Part model, mm, in its own coordinate system. Face numbers are marked on the shaded views. A direction names the side the tool comes from. Give positions to 0.01 mm unless a question says otherwise; leave off trailing zeros. Write each loop counter-clockwise with the first axis right and the second up, starting at its lowest first coordinate (ties: lowest second). Pieces come first, ordered by that corner, then holes.
```python
from build123d import *

# Parameters (mm, degrees)
SKETCH_1_R          = 20
SKETCH_1_W          = 63.973509934
SKETCH_1_H          = 26
EXTRUDE_1_DEPTH     = 10
SKETCH_2_W          = 45
SKETCH_2_H          = 20
CUT_EXTRUDE_1_DEPTH = 7
SKETCH_3_R          = 10
CUT_EXTRUDE_2_DEPTH = 8
SKETCH_4_R          = 4
CUT_EXTRUDE_3_DEPTH = 7
SKETCH_6_W          = 10
SKETCH_6_H          = 8
EXTRUDE_2_DEPTH     = 15
CHAMFER_2_SIZE      = 5
EXTRUDE_3_DEPTH     = 20
SKETCH_8_W          = 10
SKETCH_8_H          = 12.77482578
EXTRUDE_4_DEPTH     = 15
SKETCH_9_W          = 7
SKETCH_9_H          = 20
EXTRUDE_5_DEPTH     = 10
SKETCH_10_W         = 7
SKETCH_10_H         = 20
EXTRUDE_6_DEPTH     = 7
SKETCH_11_W         = 10
SKETCH_11_H         = 15
CUT_EXTRUDE_5_DEPTH = 60.88841868
SKETCH_12_W         = 10
SKETCH_12_H         = 18
SKETCH_12_H_2       = 20.77482578
EXTRUDE_7_DEPTH     = 15
CUT_EXTRUDE_6_DEPTH = 15
FILLET_1_R          = 1
CHAMFER_3_SIZE      = 1
FILLET_2_R          = 2
SKETCH_14_R         = 7.5
SKETCH_14_R_2       = 4
EXTRUDE_8_DEPTH     = 2
FILLET_3_R          = 2
SKETCH_16_R         = 2.5
CUT_EXTRUDE_7_DEPTH = 3
CHAMFER_4_SIZE      = 0.5
FILLET_4_R          = 2


# Some blends are built 0.0001 mm under size
with BuildPart() as part:
    # 草图1 → 凸台-拉伸1 (new body)
    with BuildSketch(Plane(origin=(0, 0, 0), x_dir=(0, 0, -1), z_dir=(1, 0, 0))):
        with Locations((31.986754967, 0)):
            Circle(SKETCH_1_R)
        Rectangle(SKETCH_1_W, SKETCH_1_H)
    extrude(amount=EXTRUDE_1_DEPTH)

    # 草图2 → 切除-拉伸1 (cut)
    with BuildSketch(Plane(origin=(10, 0, 0), x_dir=(0, 0, -1), z_dir=(1, 0, 0))):
        with Locations((-9.486754967, 0)):
            Rectangle(SKETCH_2_W, SKETCH_2_H)
    extrude(amount=-CUT_EXTRUDE_1_DEPTH, mode=Mode.SUBTRACT)

    # 草图3 → 切除-拉伸2 (cut)
    with BuildSketch(Plane(origin=(10, 0, 0), x_dir=(0, 0, -1), z_dir=(1, 0, 0))):
        with Locations((31.986754967, 0)):
            Circle(SKETCH_3_R)
    extrude(amount=-CUT_EXTRUDE_2_DEPTH, mode=Mode.SUBTRACT)

    # 草图4 → 切除-拉伸3 (cut)
    with BuildSketch(Plane(origin=(2, 0, 0), x_dir=(0, 0, -1), z_dir=(1, 0, 0))):
        with Locations((31.986754967, 0)):
            Circle(SKETCH_4_R)
    extrude(amount=-CUT_EXTRUDE_3_DEPTH, mode=Mode.SUBTRACT)

    # 草图6 → 凸台-拉伸2 (add)
    with BuildSketch(Plane.XZ.offset(13)):
        with Locations((5, -12.788070813)):
            Rectangle(SKETCH_6_W, SKETCH_6_H)
        with Locations((5, 27.986754967)):
            Rectangle(SKETCH_6_W, SKETCH_6_H)
    extrude(amount=EXTRUDE_2_DEPTH)

    # 倒角2
    # the kernel refuses this chamfer: 5, 3.546264764 mm, written as the material it adds along each edge
    with BuildSketch(Plane(origin=(10, -13, -16.788070813), x_dir=(0, -0.6995038411281902, -0.7146288381019251), z_dir=(-1, 0, 0))) as chamfer_2_piece_1:
        with BuildLine():
            Line((3.535736125, 0), (CHAMFER_2_SIZE * 0.699503841128, CHAMFER_2_SIZE * 0.714628838102))
            Line((CHAMFER_2_SIZE * 0.699503841128, CHAMFER_2_SIZE * 0.714628838102), (0, 0))
            ThreePointArc((0, 0), (1.768947181, 0.07828713), (3.535736125, 0))
        make_face()
    extrude(amount=10)

    # 草图7 → 凸台-拉伸3 (add)
    with BuildSketch(Plane.XY.offset(31.986754967)):
        Polygon((3, -10), (3, 10), (10, 10), (10, 13), (0, 13), (0, -28), (10, -28), (10, -10), align=None)
    extrude(amount=EXTRUDE_3_DEPTH)

    # 草图8 → 凸台-拉伸4 (add)
    with BuildSketch(Plane.XZ.offset(13)):
        with Locations((5, -2.400657923)):
            Rectangle(SKETCH_8_W, SKETCH_8_H)
    extrude(amount=EXTRUDE_4_DEPTH)

    # 草图9 → 凸台-拉伸5 (add)
    with BuildSketch(Plane.XY.offset(-13.013245033)):
        with Locations((6.5, 0)):
            Rectangle(SKETCH_9_W, SKETCH_9_H)
    extrude(amount=EXTRUDE_5_DEPTH)

    # 草图10 → 凸台-拉伸6 (add)
    with BuildSketch(Plane.XY.offset(-3.013245033)):
        with Locations((6.5, 0)):
            Rectangle(SKETCH_10_W, SKETCH_10_H)
    extrude(amount=EXTRUDE_6_DEPTH)

    # 草图11 → 切除-拉伸5 (cut, through all)
    with BuildSketch(Plane(origin=(10, 0, 0), x_dir=(0, 0, -1), z_dir=(1, 0, 0))):
        with Locations((-46.986754967, -20.5)):
            Rectangle(SKETCH_11_W, SKETCH_11_H)
    extrude(amount=-CUT_EXTRUDE_5_DEPTH, mode=Mode.SUBTRACT)

    # 草图12 → 凸台-拉伸7 (add)
    with BuildSketch(Plane.XZ.offset(28)):
        with Locations((5, 32.986754967)):
            Rectangle(SKETCH_12_W, SKETCH_12_H)
        with Locations((5, -6.400657923)):
            Rectangle(SKETCH_12_W, SKETCH_12_H_2)
    extrude(amount=EXTRUDE_7_DEPTH)

    # 草图13 → 切除-拉伸6 (cut)
    with BuildSketch(Plane.ZY):
        Polygon((-11.611311333, -29.697810406), (-0.558833166, -29.697810406), (-6.085072249, -39.916139278), align=None)
        Polygon((-6.085072249, -14.886974177), (-11.611311333, -25.105303048), (-0.558833166, -25.105303048), align=None)
        Polygon((38.707104745, -25.105303048), (27.654626578, -25.105303048), (33.180865662, -14.886974177), align=None)
        Polygon((33.180865662, -39.916139278), (38.707104745, -29.697810406), (27.654626578, -29.697810406), align=None)
    extrude(amount=-CUT_EXTRUDE_6_DEPTH, mode=Mode.SUBTRACT)

    # 圆角1
    fillet_1_edges = [part.edges().sort_by_distance(p)[0] for p in [
        (5, -39.916139278, 33.180865662),
        (5, -29.697810406, 27.654626578),
        (5, -29.697810406, 38.707104745),
        (5, -14.886974177, 33.180865662),
        (5, -25.105303048, 38.707104745),
        (5, -25.105303048, 27.654626578),
        (5, -14.886974177, -6.085072249),
        (5, -25.105303048, -0.558833166),
        (5, -25.105303048, -11.611311333),
        (5, -39.916139278, -6.085072249),
        (5, -29.697810406, -11.611311333),
        (5, -29.697810406, -0.558833166),
    ]]
    fillet(fillet_1_edges, radius=FILLET_1_R)

    # 倒角3
    chamfer_3_edges = [part.edges().sort_by_distance(p)[0] for p in [
        (5, -43, 41.986754967),
        (5, -43, 23.986754967),
        (5, -43, 3.986754967),
        (5, -43, -16.788070813),
    ]]
    chamfer(chamfer_3_edges, length=CHAMFER_3_SIZE)

    # 圆角2
    fillet_2_edges = [part.edges().sort_by_distance(p)[0] for p in [
        (5, -13, 3.986754967),
        (5, -13, 23.986754967),
    ]]
    fillet(fillet_2_edges, radius=FILLET_2_R)

    # 草图14 → 凸台-拉伸8 (add)
    with BuildSketch(Plane.ZY):
        with Locations(Location((-31.986754967, 0, 0), (0, 0, 180))):
            Circle(SKETCH_14_R)
        with Locations(Location((-31.986754967, 0, 0), (0, 0, 180))):
            Circle(SKETCH_14_R_2, mode=Mode.SUBTRACT)
    extrude(amount=EXTRUDE_8_DEPTH)

    # 圆角3
    fillet_3_edges = [part.edges().sort_by_distance(p)[0] for p in [
        (-2, 0, -24.486754967),
    ]]
    fillet(fillet_3_edges, radius=FILLET_3_R - 0.0001)  # a hair under: the kernel refuses the full size

    # 草图16 → 切除-拉伸7 (cut)
    with BuildSketch(Plane(origin=(3, 0, 0), x_dir=(0, 0, -1), z_dir=(1, 0, 0))):
        with Locations((-43.986754967, 0)):
            Circle(SKETCH_16_R)
        with Locations((-28.986754967, 0)):
            Circle(SKETCH_16_R)
        with Locations((-13.986754967, 0)):
            Circle(SKETCH_16_R)
    extrude(amount=-CUT_EXTRUDE_7_DEPTH, mode=Mode.SUBTRACT)

    # 倒角4
    chamfer_4_edges = [part.edges().sort_by_distance(p)[0] for p in [
        (0, 0, 46.486754967),
        (0, 0, 31.486754967),
        (0, 0, 16.486754967),
    ]]
    chamfer(chamfer_4_edges, length=CHAMFER_4_SIZE)

    # 圆角4
    fillet_4_edges = [part.edges().sort_by_distance(p)[0] for p in [
        (0, 13, 17.599342077),
        (0, 1.767868063, -51.908467808),
    ]]
    fillet(fillet_4_edges, radius=FILLET_4_R)


solid = part.part
```
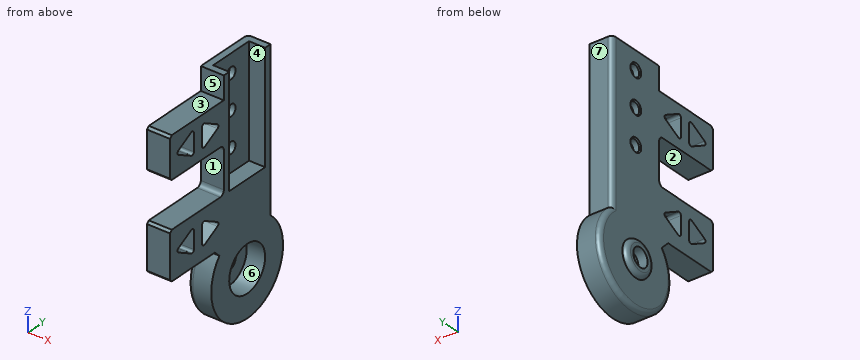
1) Wall check: L1, parallel to Z at x = 5.25, y = -28; L2, parallel to Y at x = 5.5, z = 46; L3, parallel to Y at x = 5.5, z = 28.5. Give the ranges that are in metal, low to high.
Answers follow:
L1: z = -16.79 to 3.99, 23.99 to 41.99
L2: y = -13 to -10, 10 to 13
L3: y = -43 to -31.26, -30.14 to -24.66, -23.54 to -10, 10 to 13
2) Two-plate mould, pull along Z, no slides. Class the marked faces 1, 2, 3 and 4: +Z half, -Z half, draft (parallel to the pull), parting line (faces both ways), or undercut.
Answers follow:
face 1: undercut
face 2: undercut
face 3: +Z half
face 4: draft
3) 3-axis set-ups, long thin cutter, end or side, ignore diameter. For the marked faces 5, 6 and 7: which of +Z, -Z, +X, -X, +Y, -Y reach the whole face in a straight line?
Answers follow:
face 5: +Z, +X, -X, -Y
face 6: +X
face 7: +Z, +X, -X, +Y
4) Saw through at C-C, the plane y = -36. Write the cut outline in (x, z).
Answers follow:
outline: (0, -16.79) - (10, -16.79) - (10, -8.2) - (0, -8.2) - close; (0, -3.97) - (10, -3.97) - (10, 3.99) - (0, 3.99) - close; (0, 23.99) - (10, 23.99) - (10, 31.06) - (0, 31.06) - close; (0, 35.3) - (10, 35.3) - (10, 41.99) - (0, 41.99) - close
5) Saw through at A-A, the plane z = 19. Write the cut outline in (x, y).
Answers follow:
outline: (0, -13) - (10, -13) - (10, -10) - (3, -10) - (3, 10) - (10, 10) - (10, 13) - (2, 13) arc R2 ccw to (0, 11) - close
6) Saw through at B-B, the plane y = 0. Count the separate pieces of the cut face and the enclosed holes in it, then the cut area to 3 significant figures.
Answers follow:
separate pieces: 5
enclosed holes: 0
area: 493 mm2
7) Pin check, flat tips, straight feed: pin 1 Ø2 at (x, z) = (5, 38.5) entering from +Y; pin 2 Ø2 at (x, y) = (1, -32.5) entering from -Z; pin 3 Ø6 at (y, z) = (1.5, 38.5) entering from +X; pin 4 Ø4.5 at (y, z) = (0, 28.99) entering from -X. Stop position of each tip, or through.
Answers follow:
pin 1: stops at y = 13
pin 2: stops at z = -16.79
pin 3: stops at x = 3
pin 4: passes through
